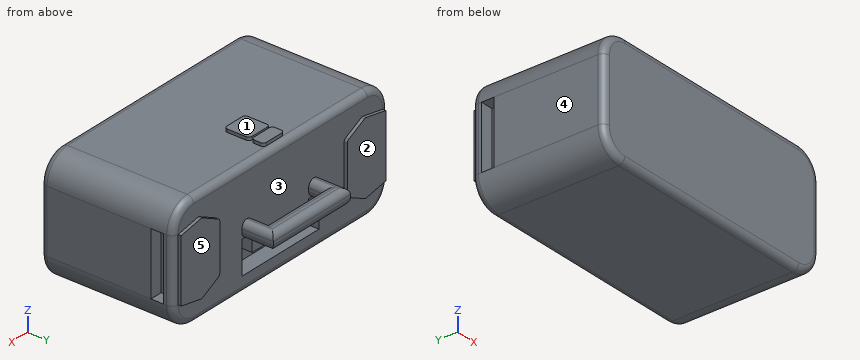
from build123d import *

# Parameters (mm, degrees)
SKIZZE1_W                       = 418
SKIZZE1_H                       = 210
AUFSATZ_LINEAR_AUSTRAGEN1_DEPTH = 90
VERRUNDUNG1_R                   = 40
SCHNITT_LINEAR_AUSTRAGEN1_DEPTH = 25
AUFSATZ_LINEAR_AUSTRAGEN2_DEPTH = 12.5
VERRUNDUNG2_R                   = 10
SKIZZE5_W                       = 100
SKIZZE5_H                       = 20
SCHNITT_LINEAR_AUSTRAGEN2_DEPTH = 20
SKIZZE6_W                       = 100
SKIZZE6_H                       = 20
SCHNITT_LINEAR_AUSTRAGEN3_DEPTH = 20
VERRUNDUNG4_R                   = 10
AUFSATZ_LINEAR_AUSTRAGEN3_DEPTH = 5
AUFSATZ_LINEAR_AUSTRAGEN4_DEPTH = 5


with BuildPart() as part:
    # Skizze1 → Aufsatz-Linear austragen1 (new, symmetric)
    with BuildSketch(Plane.XY):
        with Locations((0, 105)):
            Rectangle(SKIZZE1_W, SKIZZE1_H)
    extrude(amount=AUFSATZ_LINEAR_AUSTRAGEN1_DEPTH, both=True)

    # Verrundung1
    verrundung1_edges = [part.edges().sort_by_distance(p)[0] for p in [
        (209, 105, 90),
        (-209, 105, 90),
        (209, 105, -90),
        (-209, 105, -90),
    ]]
    fillet(verrundung1_edges, radius=VERRUNDUNG1_R)

    # Skizze3 → Schnitt-Linear austragen1 (cut)
    with BuildSketch(Plane(origin=(0, 210, 0), x_dir=(1, 0, 0), z_dir=(0, 1, 0))):
        Polygon((-75, -10), (-75, 65), (75, 65), (75, -10), (55, -10), (55, 40), (-55, 40), (-55, -10), align=None)
    extrude(amount=-SCHNITT_LINEAR_AUSTRAGEN1_DEPTH, mode=Mode.SUBTRACT)

    # Skizze4 → Aufsatz-Linear austragen2 (add, symmetric)
    with BuildSketch(Plane.XY):
        Polygon((-75, 185), (-75, 260), (75, 260), (75, 185), (55, 185), (55, 235), (-55, 235), (-55, 185), align=None)
    extrude(amount=AUFSATZ_LINEAR_AUSTRAGEN2_DEPTH, both=True)

    # Verrundung2
    verrundung2_edges = [part.edges().sort_by_distance(p)[0] for p in [
        (-75, 235, -12.5),
        (-55, 222.5, -12.5),
        (55, 222.5, -12.5),
        (0, 235, -12.5),
        (0, 260, -12.5),
        (75, 235, -12.5),
        (75, 235, 12.5),
        (55, 222.5, 12.5),
        (0, 260, 12.5),
        (0, 235, 12.5),
        (-55, 222.5, 12.5),
        (-75, 235, 12.5),
    ]]
    fillet(verrundung2_edges, radius=VERRUNDUNG2_R - 0.0001)  # a hair under: the kernel refuses the full size

    # Skizze5 → Schnitt-Linear austragen2 (cut)
    with BuildSketch(Plane(origin=(209, 0, 0), x_dir=(0, 0, -1), z_dir=(1, 0, 0))):
        with Locations((0, 185)):
            Rectangle(SKIZZE5_W, SKIZZE5_H)
    extrude(amount=-SCHNITT_LINEAR_AUSTRAGEN2_DEPTH, mode=Mode.SUBTRACT)

    # Skizze6 → Schnitt-Linear austragen3 (cut)
    with BuildSketch(Plane.ZY.offset(209)):
        with Locations((0, 185)):
            Rectangle(SKIZZE6_W, SKIZZE6_H)
    extrude(amount=-SCHNITT_LINEAR_AUSTRAGEN3_DEPTH, mode=Mode.SUBTRACT)

    # Verrundung4
    verrundung4_edges = [part.edges().sort_by_distance(p)[0] for p in [
        (0, 0, 90),
        (0, 210, 90),
        (0, 210, -90),
        (-209, 210, 0),
        (209, 210, 0),
        (-197.284271247, 210, 78.284271247),
        (-197.284271247, 210, -78.284271247),
        (197.284271247, 210, -78.284271247),
        (197.284271247, 210, 78.284271247),
        (209, 0, 0),
        (0, 0, -90),
        (-209, 0, 0),
        (-197.284271247, 0, 78.284271247),
        (-197.284271247, 0, -78.284271247),
        (197.284271247, 0, -78.284271247),
        (197.284271247, 0, 78.284271247),
    ]]
    fillet(verrundung4_edges, radius=VERRUNDUNG4_R)

    # Skizze7 → Aufsatz-Linear austragen3 (add)
    with BuildSketch(Plane(origin=(0, 210, 0), x_dir=(1, 0, 0), z_dir=(0, 1, 0))):
        with BuildLine():
            Line((-199, 50), (-160.65313505, 57.190037178))
            ThreePointArc((-160.65313505, 57.190037178), (-159.038186315, 57.227347612), (-157.495624397, 56.747812198))
            Line((-157.495624397, 56.747812198), (-126.763932023, 41.381966011))
            ThreePointArc((-126.763932023, 41.381966011), (-124.746745958, 39.538485617), (-124, 36.909830056))
            Line((-124, 36.909830056), (-124, -36.909830056))
            ThreePointArc((-124, -36.909830056), (-124.746745958, -39.538485617), (-126.763932023, -41.381966011))
            Line((-126.763932023, -41.381966011), (-157.495624397, -56.747812198))
            ThreePointArc((-157.495624397, -56.747812198), (-159.038186315, -57.227347612), (-160.65313505, -57.190037178))
            Line((-160.65313505, -57.190037178), (-199, -50))
            Line((-199, -50), (-199, 50))
        make_face()
        with BuildLine():
            Line((199, 50), (199, -50))
            Line((199, -50), (160.65313505, -57.190037178))
            ThreePointArc((160.65313505, -57.190037178), (159.038186315, -57.227347612), (157.495624397, -56.747812198))
            Line((157.495624397, -56.747812198), (126.763932023, -41.381966011))
            ThreePointArc((126.763932023, -41.381966011), (124.746745958, -39.538485617), (124, -36.909830056))
            Line((124, -36.909830056), (124, 36.909830056))
            ThreePointArc((124, 36.909830056), (124.746745958, 39.538485617), (126.763932023, 41.381966011))
            Line((126.763932023, 41.381966011), (157.495624397, 56.747812198))
            ThreePointArc((157.495624397, 56.747812198), (159.038186315, 57.227347612), (160.65313505, 57.190037178))
            Line((160.65313505, 57.190037178), (199, 50))
        make_face()
    extrude(amount=AUFSATZ_LINEAR_AUSTRAGEN3_DEPTH)

    # Skizze8 → Aufsatz-Linear austragen4 (add)
    with BuildSketch(Plane.XY.offset(90)):
        with BuildLine():
            Line((-15, 200), (15, 200))
            ThreePointArc((15, 200), (18.535533906, 198.535533906), (20, 195))
            Line((20, 195), (20, 185))
            ThreePointArc((20, 185), (18.535533906, 181.464466094), (15, 180))
            Line((15, 180), (-15, 180))
            ThreePointArc((-15, 180), (-18.535533906, 181.464466094), (-20, 185))
            Line((-20, 185), (-20, 195))
            ThreePointArc((-20, 195), (-18.535533906, 198.535533906), (-15, 200))
        make_face()
        with BuildLine():
            Line((-15, 177), (15, 177))
            ThreePointArc((15, 177), (18.535533906, 175.535533906), (20, 172))
            Line((20, 172), (20, 142))
            ThreePointArc((20, 142), (18.535533906, 138.464466094), (15, 137))
            Line((15, 137), (-15, 137))
            ThreePointArc((-15, 137), (-18.535533906, 138.464466094), (-20, 142))
            Line((-20, 142), (-20, 172))
            ThreePointArc((-20, 172), (-18.535533906, 175.535533906), (-15, 177))
        make_face()
    extrude(amount=AUFSATZ_LINEAR_AUSTRAGEN4_DEPTH)


solid = part.part
Part model, mm, in its own coordinate system. Face numbers are marked on the shaded views. A direction names the side the tool comes from. Give positions to 0.01 mm unless a question says otherwise; leave off trailing zeros. Order: outer loops, then holes, each group sorted by start corner. A loop starts at its lowest first (then second) coordinate and runs counter-clockwise, first axis right, second up. Notation, with made-up numbers: (73, -13) - (90, -13) arc R9 cw to (90, 3) - close; hole circle Ø7 at (69.5, 36). An arc over 180 degrees is marked (long way). Use a Markdown table: item, result.
1) Saw through at C-C on y = 77.5. List the corners of the cut face in (x, z), plus the area to 3 significant figures.
Checked values:
| item | result |
|---|---|
| outline | (-209, -50) arc R40 ccw to (-169, -90) - (169, -90) arc R40 ccw to (209, -50) - (209, 50) arc R40 ccw to (169, 90) - (-169, 90) arc R40 ccw to (-209, 50) - close |
| area | 73,900 mm² |
2) 3-axis set-ups, long thin cutter, end or side, ignore diameter. For the marked faces 1 and 2: which of +Z, -Z, +X, -X, +Y, -Y reach the whole face in a straight line?
Checked values:
| item | result |
|---|---|
| face 1 | +Z, +X, -X, +Y, -Y |
| face 2 | +Z, -Z, -X, +Y |
3) Two-plate mould, pull along X, no slides. Class the marked faces 3, 4 and 5: +X half, -X half, draft (parallel to the pull), parting line (faces both ways), or undercut.
Checked values:
| item | result |
|---|---|
| face 3 | undercut |
| face 4 | -X half |
| face 5 | draft |
4) Saw through at A-A on x = -10.5. List the corners of the cut face in (y, z).
Checked values:
| item | result |
|---|---|
| outline | (0, -80) arc R10 ccw to (10, -90) - (200, -90) arc R10 ccw to (210, -80) - (210, -65) - (185, -65) - (185, -40) - (210, -40) - (210, 80) arc R10 ccw to (200, 90) - (200, 95) - (180, 95) - (180, 90) - (177, 90) - (177, 95) - (137, 95) - (137, 90) - (10, 90) arc R10 ccw to (0, 80) - close; (235, -2.5) arc R10 ccw to (245, -12.5) - (250, -12.5) arc R10 ccw to (260, -2.5) - (260, 2.5) arc R10 ccw to (250, 12.5) - (245, 12.5) arc R10 ccw to (235, 2.5) - close |
5) Saw through at B-B on z = 26.5. List the corners of the cut face in (x, y), plus the area to 3 significant figures.
Checked values:
| item | result |
|---|---|
| outline | (-209, 10) arc R10 ccw to (-199, 0) - (199, 0) arc R10 ccw to (209, 10) - (209, 175) - (189, 175) - (189, 195) - (209, 195) - (209, 200) arc R10 ccw to (199, 210) - (199, 215) - (124, 215) - (124, 210) - (-124, 210) - (-124, 215) - (-199, 215) - (-199, 210) arc R10 ccw to (-209, 200) - (-209, 195) - (-189, 195) - (-189, 175) - (-209, 175) - close |
| area | 87,600 mm² |
6) Probe L1, parallel to Y at x = 138, z = -45; L2, parallel to Z at x = -104.5, y = 35; L3, parallel to Y at x = -53, z = 69.5. List the from-to ranges inside material, lowest first. Write a range as from..to.
Checked values:
| item | result |
|---|---|
| L1 | 0..215 |
| L2 | -90..90 |
| L3 | 0..210 |
7) Saw through at D-D on x = -97.5. List the corners of the cut face in (y, z), plus the area to 3 significant figures.
Checked values:
| item | result |
|---|---|
| outline | (0, -80) arc R10 ccw to (10, -90) - (200, -90) arc R10 ccw to (210, -80) - (210, 80) arc R10 ccw to (200, 90) - (10, 90) arc R10 ccw to (0, 80) - close |
| area | 37,700 mm² |
8) Flat gauge pins, fed straight in: P1, Ø16, axis at x = 201, y = 181.5, coming from the +Z side; P2, Ø1.5, axis at x = 50.5, y = 202.5, coming from the -Z side; P3, Ø4, axis at x = 165.5, z = -6, coming from the +Y side. Where does each tip first touch, or does it go through?
Checked values:
| item | result |
|---|---|
| P1 | z = 82 |
| P2 | z = -89.85 |
| P3 | y = 215 |
